The model under review builds one solid part; all positions refer to its coordinate system, in mm. Face numbers are marked on the shaded views. A direction names the side the tool comes from. Round coordinates to 2 decimals unless told otherwise and drop trailing zeros. Write each loop counter-clockwise with the first axis right and the second up, starting at its lowest first coordinate (ties: lowest second). Pieces come first, ordered by that corner, then holes. Notation, with made-up numbers: (-31, 61) -> (15, 61) arc R14 cw to (15, 72) -> close; hole circle Ø9 at (68.25, -31.5). An arc over 180 degrees is marked (long way). Answer as a JSON object with one key per item and string values. Group by question number.
1) We need section B-B, the plane y = -19.5. Write out the cut boundary in (x, z), then the cut area to 3 significant figures.
2) Insertion check: pin 1 Ø5 at (y, z) = (13.36, 0) entering from -X; pin 2 Ø1 at (x, z) = (-2.5, 4.5) entering from +Y; pin 3 Ø3 at (x, z) = (-2.5, 5.5) entering from -Y; pin 4 Ø3.5 at (x, y) = (0, -21.14) entering from -Z. Each pin has a flat end and moves straight along its axis. Give the tip position at first contact, or say it passes through.
3) We need section D-D, the plane z = 7.75. Write out the cut boundary in (x, y).
4) Machinability: for the marked faces 1, 2, 3, 4 and 5, which of the approach directions +Z, -Z, +X, -X, +Y, -Y give a long, thin tool a straight path to every point of the face, cutting with its end or side? Answer none if there is none.
5) We need section A-A, the plane z = 6. Write out the cut boundary in (x, y), then the cut area to 3 significant figures.
6) Mouldability with a two-part tool opening along Y and no side actions: class the marked faces 6, 7 and 8 as pulls with the +Y half, pulls with the -Y half, needs draft (parallel to the pull), parting line crosses it, or undercut.
7) We need section C-C, the plane x = 0. Count the separate pieces of the cut face and the enclosed holes in it, then the cut area to 3 significant figures.
8) To check wall thickness, follow probe 1 along Z at (x, y) = (0, -3.2); probe 2 along X at (y, z) = (11.5, 2); probe 3 along Y at (x, z) = (0, -2.2). State the ranges of each line that lie inside material, in increasing order. Write a range as [from, to].
from build123d import *

# Parameters (mm, degrees)
F1_DEPTH     = 1.5
F2_R         = 2
F3_DEPTH     = 3.001
F6_DEPTH     = 30
F7_W         = 14.9228225192
F7_H         = 3.5
F8_DEPTH     = 12.5
F9_W         = 7
F9_H         = 3
F10_DEPTH    = 8.5
F11_R        = 2
F12_DEPTH    = 12.5
F13_R        = 1
F14_DEPTH    = 21.001
F15_T1_DEPTH = 11.2055438024


# Not quite as in the source:
# - a fillet or chamfer that OpenCascade refuses, or shapes differently, is made with other operations: its cross-section is extruded or revolved along the edge and cut away or added


with BuildPart() as f1:
    # F0 (on Right) → F1 (new body, symmetric)
    with BuildSketch(Plane.YZ):
        Polygon((16.8634157784, -1.1044778318), (16.8634157784, 0.8955221682), (14.8634157784, 2.8955221682), (8.8634157784, 2.8955221682), (6.8634157784, 0.8955221682), (6.8634157784, -1.1044778318), (8.8634157784, -3.1044778318), (14.8634157784, -3.1044778318), align=None)
    extrude(amount=F1_DEPTH, both=True)

    # F2 (on face) → F3 (cut, through all)
    with BuildSketch(Plane(origin=(-1.5, 0, 0), x_dir=(0, -1, 0), z_dir=(-1, 0, 0))):
        with Locations((-13.3634157784, 0)):
            Circle(F2_R)
    extrude(amount=-F3_DEPTH, mode=Mode.SUBTRACT)

    # F4 (on Top) → F5 (revolve)
    with BuildSketch(Plane.XY):
        Polygon((0, 4.8634157784), (0, 9.8634157784), (-1.5, 9.8634157784), (-3.5, 4.8634157784), align=None)
    revolve(axis=Axis((0, 7.3634157784, 0), (0, 1, 0)))

    # F6 (add): a face of the model
    f6_faces = [f1.faces().sort_by_distance(p)[0] for p in [
        (0, 4.8634157784, 0),
    ]]
    extrude(f6_faces, amount=F6_DEPTH)

    # F7 (on Right) → F8 (cut, symmetric)
    with BuildSketch(Plane.YZ):
        with Locations((-23.5979954812, 0)):
            Rectangle(F7_W, F7_H)
    extrude(amount=F8_DEPTH, both=True, mode=Mode.SUBTRACT)

    # F9 (on Top) → F10 (join)
    with BuildSketch(Plane.XY):
        with Locations((0, -2.6365842216)):
            Rectangle(F9_W, F9_H)
    extrude(amount=F10_DEPTH)

    # F11 (on Top) → F12 (cut, symmetric)
    with BuildSketch(Plane.XY):
        with Locations((0, -21.1365842216)):
            Circle(F11_R)
    extrude(amount=F12_DEPTH, both=True, mode=Mode.SUBTRACT)

    # F13 (on face) → F14 (cut, through all)
    with BuildSketch(Plane.XZ.offset(4.1365842216)):
        with Locations((0, 6)):
            Circle(F13_R)
    extrude(amount=-F14_DEPTH, mode=Mode.SUBTRACT)

    # F15: chamfer of 1 on 2 edges, made by hand

    # F15_s2 → F15_t1 (cut)
    with BuildSketch(Plane.YZ.offset(-5.6027719012)):
        Polygon((-24.1365842216, -1.75), (-25.1365842216, -2.75), (-25.1365842216, -1.75), align=None)
        Polygon((-24.1365842216, 1.75), (-25.1365842216, 2.75), (-25.1365842216, 1.75), align=None)
    extrude(amount=F15_T1_DEPTH, mode=Mode.SUBTRACT)


solid = f1.part
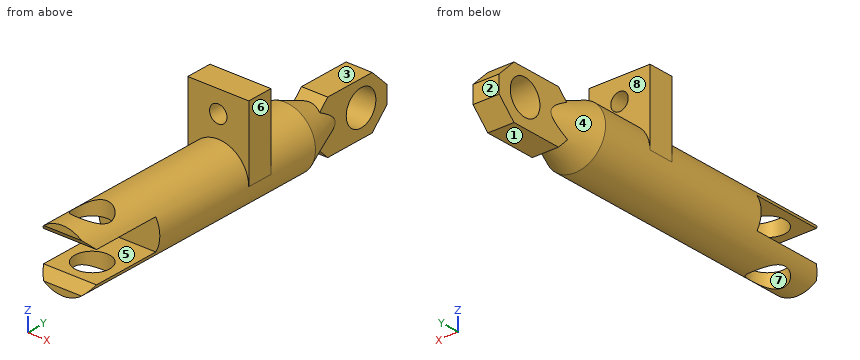
Here are the results:
{
 "1": {"outline": "(-3.03, -1.75) arc R3.5 ccw to (-1.15, -3.31) -> (-1.15, -1.75) -> close; (-3.03, 1.75) -> (-1.15, 1.75) -> (-1.15, 3.31) arc R3.5 ccw to start; (1.15, -3.31) arc R3.5 ccw to (3.03, -1.75) -> (1.15, -1.75) -> close; (1.15, 1.75) -> (3.03, 1.75) arc R3.5 ccw to (1.15, 3.31) -> close", "area": "7.29 mm^2"},
 "2": {"pin 1": "stops at x = -1.5", "pin 2": "stops at y = -1.14", "pin 3": "stops at y = -4.14", "pin 4": "passes through"},
 "3": {"outline": "(-3.5, -4.14) -> (3.5, -4.14) -> (3.5, -1.14) -> (-3.5, -1.14) -> close"},
 "4": {"face 1": "-Z, +X, -X, +Y", "face 2": "+Z, -Z, +X, -X, +Y", "face 3": "+Z, +X, -X, +Y", "face 4": "none", "face 5": "+X, -X, -Y"},
 "5": {"outline": "(-3.5, -4.14) -> (-1, -4.14) -> (-1, -1.14) -> (-3.5, -1.14) -> close; (1, -4.14) -> (3.5, -4.14) -> (3.5, -1.14) -> (1, -1.14) -> close", "area": "15.0 mm^2"},
 "6": {"face 6": "needs draft", "face 7": "undercut", "face 8": "pulls with the +Y half"},
 "7": {"separate pieces": "4", "enclosed holes": "1", "area": "226 mm^2"},
 "8": {"probe 1": "z = [-3.5, 5], [7, 8.5]", "probe 2": "x = [-1.5, 1.5]", "probe 3": "y = [-24.59, -23.14], [-19.14, 15.77]"}
}
